For this review, take the finished solid that the model builds, in its own axes (mm). Round coordinates to 2 decimals unless told otherwise and drop trailing zeros. Order: outer loops, then holes, each group sorted by start corner. A loop starts at its lowest first (then second) coordinate and runs counter-clockwise, first axis right, second up. Notation, with made-up numbers: (85.5, 65.25) - (104.5, 65.25) arc R35 ccw to (104.5, 98.25) - close; hole circle Ø5 at (81, 9). An arc over 180 degrees is marked (long way). One line per item, written item: value.
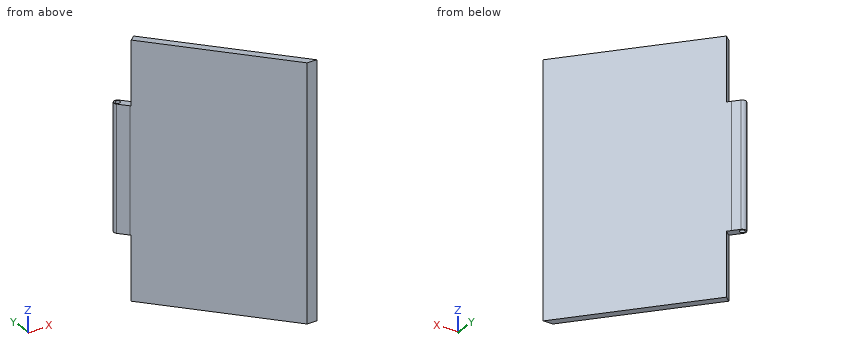
Autodesk Inventor part; units mm, degrees
ref_plane "YZ Plane" through (0, 0, 0) normal (1, 0, 0) x (0, 1, 0)
ref_plane "XZ Plane" through (0, 0, 0) normal (0, 1, 0) x (-1, 0, 0)
ref_plane "XY Plane" through (0, 0, 0) normal (0, 0, 1) x (1, 0, 0)
sketch "Эскиз1" plane through (0, 0, 0) normal (0, 0, 1) x (1, 0, 0)
  line L0 (0, 0) -> (-40.6757, 46.792)
  line L1 (-40.6757, 46.792) -> (-85.6757, 46.792)
  line L2 (-85.6757, 49.792) -> (-39.3085, 49.792)
  line L3 (-39.3085, 49.792) -> (3.975, 0)
  line L4 (-40.6757, 46.792) -> (-55.8266, 64.2212)
  line L5 (0, 0) -> (15.6604, 0)
  line L6 (-15.0802, 19.6341) -> (-42.5999, 51.292)
  line L7 (-85.6757, 51.292) -> (-42.5999, 51.292)
  circle A0 centre (-42.5999, 51.292) radius 1
  line L8 (-39.3085, 49.792) -> (-42.452, 53.4081)
  line L9 (-42.452, 53.4081) -> (-44.7161, 51.44)
  line L10 (-40.6757, 46.792) -> (-40.6757, 52.792)
  line L11 (-40.6757, 52.792) -> (-44.0999, 52.792)
  line L12 (-44.0999, 52.792) -> (-44.0999, 46.792)
  line L13 (-40.6757, 46.792) -> (-38.4115, 48.7602)
  line L14 (-40.3476, 46.4146) -> (-38.0835, 48.3828)
  point P0 (-59.7086, 51.292)
  dimension "d0" = 131
  dimension "d1" = 45
  dimension "d2" = 62
  dimension "d3" = 3
  dimension "d4" = 3
  dimension "d5" = 3
  dimension "d6" = 3
  dimension "d7" = 2
  dimension "d8" = 1.5
  dimension "d9" = 1.5
  dimension "d10" = 1.5
  dimension "d17" = 0.5
extrude "Выдавливание1" add sketch "Эскиз1" along normal mid plane 49.5 contours L0 L14 L3 L5 | L0 L13 L6 L14 | L4 L2 L6 L10 | L10 L6 L13 | L6 L13 L3 L14 | L4 L12 L7 A0 L6 L2 | L10 L2 L3 L13 L6 | L6 L2 L10 | L6 A0 L7 L12 L9 L11 L8 L10 L2 | L4 L7 L12 | L10 L8 L2 | L4 L9 L12 L7 | L11 L9 L8
fillet "Сопряжение1" radius 1.5 2 edges at (-42.452, 53.4081, 0) (-44.7161, 51.44, 0)
extrude "Выдавливание2" add sketch "Эскиз1" along normal mid plane 100 contours L0 L14 L3 L5
properties part number "Cover2"
Item 1: For P1, Ø3, axis at x = -41.5, y = 49, coming from the -Z side; P2, Ø5, axis at y = 23, z = 12, coming from the -X side; P3, Ø8, axis at y = 45.5, z = -5, coming from the +X side, all flat-tipped, find the tip position at first contact; note any pin that passes through.
Returned:
P1: z = -24.75
P2: x = -22.17
P3: x = -32.1
Item 2: Take a section at C-C (x = -28). Write out the cut boundary in (y, z).
Returned:
outline: (32.21, -50) - (36.78, -50) - (36.78, 50) - (32.21, 50) - close
Item 3: Take a section at B-B (y = 44). Write out the cut boundary in (x, z).
Returned:
outline: (-38.25, -50) - (-34.27, -50) - (-34.27, 50) - (-38.25, 50) - close
Item 4: Wall thickness on line 1 (X direction, y = 13, z = 40); line 2 (Y direction, x = -17.5, z = -36.5); line 3 (X direction, y = 34, z = -27): over which ranges is each line inside the solid? List them lowest first.
Returned:
line 1: -11.3 to -7.33
line 2: 20.13 to 24.7
line 3: -29.56 to -25.58
